Read the model definition and answer for the solid it produces. Units are mm, in the model's axes. Coordinates: 2 decimals unless noted, no trailing zeros. Write each loop counter-clockwise with the first axis right and the second up, starting at its lowest first coordinate (ties: lowest second). Pieces come first, ordered by that corner, then holes. Notation, with made-up numbers: (76.5, 43.5) -> (124.5, 43.5) arc R12 cw to (124.5, 52.5) -> close; hole circle Ø9 at (89, -18). An arc over 180 degrees is marked (long way). Answer in a Markdown table with one row per item. Add a question column.
Item 1: Section B-B on y = 1.5 is taken. Count the separate pieces of the cut face and the enclosed holes in it, then the cut area to 3 significant figures.
Item 2: Given pin 1 Ø1 at (x, z) = (15, -18.5) entering from -Y; pin 2 Ø3 at (x, y) = (8, -2.5) entering from -Z; pin 3 Ø1 at (x, z) = (8, -27) entering from +Y, each flat-ended and moving along its own axis, determine where each tip first touches the part or whether it passes through.
Item 3: Section A-A on x = 12 is taken. Write down the section's boundary in (y, z), then the cut area to 3 significant figures.
Item 4: Section C-C on z = -27.5 is taken. Write down the section's boundary in (x, y), then the cut area to 3 significant figures.
Item 5: Section D-D on y = -1 is taken. Write down the section's boundary in (x, z).
Item 6: Straight lines are drawn through the part: line 1 (Z direction, x = 13.5, y = 2.25); line 2 (Z direction, x = 7, y = 1.25); line 3 (X direction, y = 0.75, z = -2). For each, find the intervals that lie inside material, in ascending order. Write a range as from..to.
Item 7: For a pull along Z with two mould halves and no side action, classify faces 1 (the face through (0, 1, -11)), 2 (the face through (27.887, 1.232, -14.362)) as +Z half, -Z half, draft (parallel to the pull), parting line (faces both ways), or undercut.
```python
from build123d import *

# Parameters (mm, degrees)
SKETCH1_W           = 31.770430493
SKETCH1_H           = 30.262813536
BOSS_EXTRUDE1_DEPTH = 2.5
SKETCH2_W           = 31.770430493
SKETCH2_H           = 12.5
BOSS_EXTRUDE2_DEPTH = 2


with BuildPart() as part:
    # Sketch1 → Boss-Extrude1 (new body)
    with BuildSketch(Plane(origin=(0, 0, 0), x_dir=(1, 0, 0), z_dir=(0, 1, 0))):
        with Locations((15.885215247, 15.131406768)):
            Rectangle(SKETCH1_W, SKETCH1_H)
        Polygon((7.547843414, 7.63328856), (4.083741799, 7.63328856), (2.351690991, 4.63328856), (4.083741799, 1.63328856), (7.547843414, 1.63328856), (9.279894221, 4.63328856), align=None, mode=Mode.SUBTRACT)
        Polygon((14.043033942, 11.38328856), (10.578932327, 11.38328856), (8.846881519, 8.38328856), (10.578932327, 5.38328856), (14.043033942, 5.38328856), (15.77508475, 8.38328856), align=None, mode=Mode.SUBTRACT)
        Polygon((20.537843414, 7.63328856), (17.073741799, 7.63328856), (15.341690991, 4.63328856), (17.073741799, 1.63328856), (20.537843414, 1.63328856), (22.269894221, 4.63328856), align=None, mode=Mode.SUBTRACT)
        Polygon((27.033033942, 11.38328856), (23.568932327, 11.38328856), (21.836881519, 8.38328856), (23.568932327, 5.38328856), (27.033033942, 5.38328856), (28.76508475, 8.38328856), align=None, mode=Mode.SUBTRACT)
        Polygon((20.537843414, 15.13328856), (17.073741799, 15.13328856), (15.341690991, 12.13328856), (17.073741799, 9.13328856), (20.537843414, 9.13328856), (22.269894221, 12.13328856), align=None, mode=Mode.SUBTRACT)
        Polygon((27.033033942, 18.88328856), (23.568932327, 18.88328856), (21.836881519, 15.88328856), (23.568932327, 12.88328856), (27.033033942, 12.88328856), (28.76508475, 15.88328856), align=None, mode=Mode.SUBTRACT)
        Polygon((20.537843414, 22.63328856), (17.073741799, 22.63328856), (15.341690991, 19.63328856), (17.073741799, 16.63328856), (20.537843414, 16.63328856), (22.269894221, 19.63328856), align=None, mode=Mode.SUBTRACT)
        Polygon((27.033033942, 26.38328856), (23.568932327, 26.38328856), (21.836881519, 23.38328856), (23.568932327, 20.38328856), (27.033033942, 20.38328856), (28.76508475, 23.38328856), align=None, mode=Mode.SUBTRACT)
        Polygon((7.547843414, 15.13328856), (4.083741799, 15.13328856), (2.351690991, 12.13328856), (4.083741799, 9.13328856), (7.547843414, 9.13328856), (9.279894221, 12.13328856), align=None, mode=Mode.SUBTRACT)
        Polygon((14.043033942, 18.88328856), (10.578932327, 18.88328856), (8.846881519, 15.88328856), (10.578932327, 12.88328856), (14.043033942, 12.88328856), (15.77508475, 15.88328856), align=None, mode=Mode.SUBTRACT)
        Polygon((7.547843414, 22.63328856), (4.083741799, 22.63328856), (2.351690991, 19.63328856), (4.083741799, 16.63328856), (7.547843414, 16.63328856), (9.279894221, 19.63328856), align=None, mode=Mode.SUBTRACT)
        Polygon((14.043033942, 26.38328856), (10.578932327, 26.38328856), (8.846881519, 23.38328856), (10.578932327, 20.38328856), (14.043033942, 20.38328856), (15.77508475, 23.38328856), align=None, mode=Mode.SUBTRACT)
    extrude(amount=BOSS_EXTRUDE1_DEPTH)

    # Sketch2 → Boss-Extrude2 (add)
    with BuildSketch(Plane.XY):
        with Locations((15.885215247, 1.25)):
            Rectangle(SKETCH2_W, SKETCH2_H)
    extrude(amount=BOSS_EXTRUDE2_DEPTH)


solid = part.part
```
Results below:
| question | item | result |
|---|---|---|
| 1 | separate pieces | 1 |
| 1 | enclosed holes | 12 |
| 1 | area | 651 mm2 |
| 2 | pin 1 | stops at y = 0 |
| 2 | pin 2 | stops at z = 0 |
| 2 | pin 3 | stops at y = 2.5 |
| 3 | outline | (-5, 0) -> (0, 0) -> (0, -5.38) -> (2.5, -5.38) -> (2.5, 0) -> (7.5, 0) -> (7.5, 2) -> (-5, 2) -> close; (0, -30.26) -> (2.5, -30.26) -> (2.5, -26.38) -> (0, -26.38) -> close; (0, -20.38) -> (2.5, -20.38) -> (2.5, -18.88) -> (0, -18.88) -> close; (0, -12.88) -> (2.5, -12.88) -> (2.5, -11.38) -> (0, -11.38) -> close |
| 3 | area | 55.7 mm2 |
| 4 | outline | (0, 0) -> (31.77, 0) -> (31.77, 2.5) -> (0, 2.5) -> close |
| 4 | area | 79.4 mm2 |
| 5 | outline | (0, 0) -> (31.77, 0) -> (31.77, 2) -> (0, 2) -> close |
| 6 | line 1 | z = -30.26..-26.38, -20.38..-18.88, -12.88..-11.38, -5.38..2 |
| 6 | line 2 | z = -30.26..-22.63, -16.63..-15.13, -9.13..-7.63, -1.63..2 |
| 6 | line 3 | x = 0..3.87, 7.76..16.86, 20.75..31.77 |
| 7 | face 1 | draft |
| 7 | face 2 | undercut |
